Check sheet for the modelled part. Datum: model origin and axes. Units: mm. Face numbers are marked on the shaded views. A direction names the side the tool comes from. Give positions to 0.01 mm unless a question says otherwise; leave off trailing zeros. Loops run counter-clockwise (first coordinate to the right, second up) from the corner with the lowest first, then second, coordinate; pieces in that order, holes last. Notation, with made-up numbers: (89.5, 65) -> (128.5, 65) arc R23 cw to (128.5, 87) -> close; hole circle Ø6 at (-16.5, -21). An arc over 180 degrees is marked (long way). Write each question's results on one line, items separated by ' | '. Start each with the question number.
1. Mould release check, pull along Z, two halves, no side actions. Record for the marked faces 1, 2, 3 and 4: +Z half, -Z half, draft (parallel to the pull), parting line (faces both ways), or undercut.
2. Cross-section at B-B on x = 10.5. Record the boundary of the cut face in (y, z).
3. Cross-section at C-C on y = 1.75. Record the boundary of the cut face in (x, z), and give its area (3 significant figures).
4. Tool access check on the marked faces 5 and 6. Record the directions out of +Z, -Z, +X, -X, +Y, -Y that give a thin tool (end or side, any length) a straight path to the whole face; none if there is none.
5. Gauge pin test, flat ends, axial feed: pin 1 Ø2 at (y, z) = (3.5, -3.5) entering from +X; pin 2 Ø1.6 at (x, z) = (8.5, -11.5) entering from +Y; pin 3 Ø10.5 at (x, z) = (3.5, 2.5) entering from +Y. Record the tip position at first contact, or that the pin passes through.
6. Cross-section at D-D on z = -2.75. Record the boundary of the cut face in (x, y), and give its area (3 significant figures).
7. Cross-section at A-A on y = 10.75. Record the boundary of the cut face in (x, z).
8. Material ranges on L1, parallel to Z at x = -4.5, y = 5.25; L2, parallel to X at y = 9.25, z = -11.5; L3, parallel to X at y = 7.5, z = -6.5, recorded low to high. Write a range as from..to.
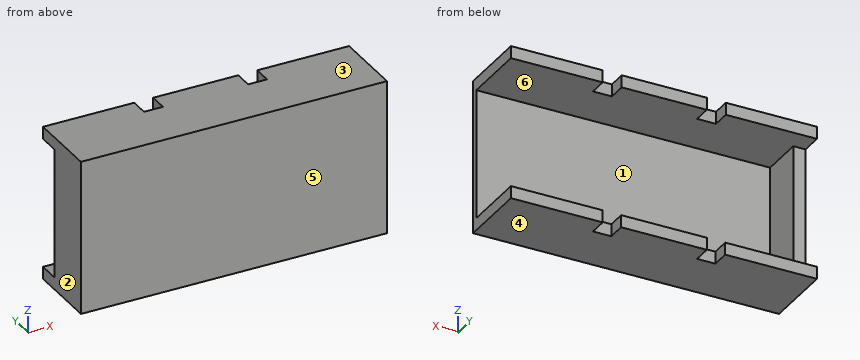
from build123d import *

# Parameters (mm, degrees)
SKETCH_1_W      = 50
SKETCH_1_H      = 25.2
EXTRUDE_1_DEPTH = 1
SKETCH_2_W      = 50
SKETCH_2_H      = 2
EXTRUDE_2_DEPTH = 7.6
SKETCH_4_W      = 15
SKETCH_4_H      = 2
SKETCH_4_W_2    = 14
EXTRUDE_3_DEPTH = 3
SKETCH_5_W      = 14.9
SKETCH_5_H      = 2
SKETCH_5_W_2    = 13.9
SKETCH_5_W_3    = 15
EXTRUDE_4_DEPTH = 3
SKETCH_6_W      = 2
SKETCH_6_H      = 25.2
EXTRUDE_5_DEPTH = 3.6
SKETCH_7_W      = 2
SKETCH_7_H      = 21.2
EXTRUDE_6_DEPTH = 3.5


with BuildPart() as part:
    # 草图1 → 凸台-拉伸1 (new body)
    with BuildSketch(Plane(origin=(0, 0, 0), x_dir=(1, 0, 0), z_dir=(0, 1, 0))):
        Rectangle(SKETCH_1_W, SKETCH_1_H)
    extrude(amount=EXTRUDE_1_DEPTH)

    # 草图2 → 凸台-拉伸2 (add)
    with BuildSketch(Plane(origin=(0, 1, 0), x_dir=(1, 0, 0), z_dir=(0, 1, 0))):
        with Locations((0, 11.6)):
            Rectangle(SKETCH_2_W, SKETCH_2_H)
        with Locations((0, -11.6)):
            Rectangle(SKETCH_2_W, SKETCH_2_H)
    extrude(amount=EXTRUDE_2_DEPTH)

    # 草图4 → 凸台-拉伸3 (add)
    with BuildSketch(Plane(origin=(0, 8.6, 0), x_dir=(1, 0, 0), z_dir=(0, 1, 0))):
        with Locations((-17.5, 11.6)):
            Rectangle(SKETCH_4_W, SKETCH_4_H)
        with Locations((0, 11.6)):
            Rectangle(SKETCH_4_W_2, SKETCH_4_H)
        with Locations((17.5, 11.6)):
            Rectangle(SKETCH_4_W, SKETCH_4_H)
    extrude(amount=EXTRUDE_3_DEPTH)

    # 草图5 → 凸台-拉伸4 (add)
    with BuildSketch(Plane(origin=(0, 8.6, 0), x_dir=(1, 0, 0), z_dir=(0, 1, 0))):
        with Locations((-17.55, -11.6)):
            Rectangle(SKETCH_5_W, SKETCH_5_H)
        with Locations((-0.05, -11.6)):
            Rectangle(SKETCH_5_W_2, SKETCH_5_H)
        with Locations((17.5, -11.6)):
            Rectangle(SKETCH_5_W_3, SKETCH_5_H)
    extrude(amount=EXTRUDE_4_DEPTH)

    # 草图6 → 凸台-拉伸5 (add)
    with BuildSketch(Plane(origin=(0, 1, 0), x_dir=(1, 0, 0), z_dir=(0, 1, 0))):
        with Locations((-24, 0)):
            Rectangle(SKETCH_6_W, SKETCH_6_H)
    extrude(amount=EXTRUDE_5_DEPTH)

    # 草图7 → 凸台-拉伸6 (add)
    with BuildSketch(Plane(origin=(0, 4.6, 0), x_dir=(1, 0, 0), z_dir=(0, 1, 0))):
        with Locations((-24, 0)):
            Rectangle(SKETCH_7_W, SKETCH_7_H)
    extrude(amount=EXTRUDE_6_DEPTH)


solid = part.part
Geometry says:
1) face 1: undercut | face 2: draft | face 3: +Z half | face 4: -Z half
2) outline: (0, -12.6) -> (11.6, -12.6) -> (11.6, -10.6) -> (1, -10.6) -> (1, 10.6) -> (11.6, 10.6) -> (11.6, 12.6) -> (0, 12.6) -> close
3) outline: (-25, -12.6) -> (25, -12.6) -> (25, -10.6) -> (-23, -10.6) -> (-23, 10.6) -> (25, 10.6) -> (25, 12.6) -> (-25, 12.6) -> close | area: 242 mm^2
4) face 5: +Z, -Z, +X, -X, -Y | face 6: +X, +Y
5) pin 1: x = -23 | pin 2: y = 8.6 | pin 3: y = 1
6) outline: (-25, 0) -> (25, 0) -> (25, 1) -> (-23, 1) -> (-23, 8.1) -> (-25, 8.1) -> close | area: 64.2 mm^2
7) outline: (-25, -12.6) -> (-10, -12.6) -> (-10, -10.6) -> (-25, -10.6) -> close; (-25, 10.6) -> (-10.1, 10.6) -> (-10.1, 12.6) -> (-25, 12.6) -> close; (-7, -12.6) -> (7, -12.6) -> (7, -10.6) -> (-7, -10.6) -> close; (-7, 10.6) -> (6.9, 10.6) -> (6.9, 12.6) -> (-7, 12.6) -> close; (10, -12.6) -> (25, -12.6) -> (25, -10.6) -> (10, -10.6) -> close; (10, 10.6) -> (25, 10.6) -> (25, 12.6) -> (10, 12.6) -> close
8) L1: -12.6..-10.6, 10.6..12.6 | L2: -25..-10, -7..7, 10..25 | L3: -25..-23
